```python
from build123d import *

# Parameters (mm, degrees)
SKETCH_W     = 84.3
SKETCH_H     = 85.3
PAD_DEPTH    = 10
SKETCH001_R  = 10
POCKET_DEPTH = 10.001


with BuildPart() as part:
    # Sketch → Pad (new body)
    with BuildSketch(Plane.XY):
        Rectangle(SKETCH_W, SKETCH_H)
    extrude(amount=PAD_DEPTH)

    # Sketch001 (on Face6 of Pad) → Pocket (cut, through all)
    with BuildSketch(Plane.XY.offset(10)):
        with Locations((12, 12.5)):
            Circle(SKETCH001_R)
        Polygon((-42.15, -32.65), (-42.15, -42.65), (-32.15, -42.65), align=None)
        with BuildLine():
            ThreePointArc((42.15, 12.50004), (33.319274, 33.819265), (12.000052, 42.65))
            Line((12.000052, 42.65), (42.15, 84.3))
            Line((42.15, 84.3), (42.15, 12.50004))
        make_face()
    extrude(amount=-POCKET_DEPTH, mode=Mode.SUBTRACT)


solid = part.part
```
Check sheet for the modelled part. Datum: model origin and axes. Units: mm. Round coordinates to 2 decimals unless told otherwise and drop trailing zeros. Order: outer loops, then holes, each group sorted by start corner. A loop starts at its lowest first (then second) coordinate and runs counter-clockwise, first axis right, second up.
1) Section check B-B (x = 3). Record the boundary of the cut face in (y, z).
2) Section check A-A (z = 3.25). Record the boundary of the cut face in (x, y).
3) Scan lines: line 1 (Y direction, x = 12, z = 6.75); line 2 (X direction, y = 7.5, z = 1.25); line 3 (Y direction, x = 19.5, z = 4.75). Record each from-to range of solid material in increasing order.
4) Mould release check, pull along X, two halves, no side actions. Record for faces 1 (the flat face through (42.15, -15, 5)), 2 (the flat face through (-1, 1, 10)), 3 (the flat face through (-37.1, -37.7, 5.1)), 4 (the cylindrical face through (9.83, 2.74, 5.07)): +X half, -X half, draft (parallel to the pull), parting line (faces both ways), or undercut.
Result:
1. outline: (-42.65, 0) - (8.14, 0) - (8.14, 10) - (-42.65, 10) - close; (16.86, 0) - (42.65, 0) - (42.65, 10) - (16.86, 10) - close
2. outline: (-42.15, -32.65) - (-32.15, -42.65) - (42.15, -42.65) - (42.15, 12.5) arc R30.15 ccw to (12, 42.65) - (-42.15, 42.65) - close; hole circle Ø20 at (12, 12.5)
3. line 1: y = -42.65 to 2.5, 22.5 to 42.65
3. line 2: x = -42.15 to 3.34, 20.66 to 42.15
3. line 3: y = -42.65 to 5.89, 19.11 to 41.7
4. face 1: +X half
4. face 2: draft
4. face 3: -X half
4. face 4: undercut
